The listing builds one solid part. Answer for the finished solid, in the listing's coordinates (mm). Round coordinates to 2 decimals unless told otherwise and drop trailing zeros. Loops run counter-clockwise (first coordinate to the right, second up) from the corner with the lowest first, then second, coordinate; pieces in that order, holes last. Notation, with made-up numbers: (-13.75, 78.25) -> (40.25, 78.25) arc R17 cw to (40.25, 93.25) -> close; hole circle Ø6 at (72.5, 43.5). An arc over 180 degrees is marked (long way). Use a Markdown table: item, result. Add a question column.
Q1. Given pin 1 Ø1.5 at (x, z) = (25.5, 2.5) entering from -Y; pin 2 Ø1.5 at (x, z) = (-12.5, 0.5) entering from -Y; pin 3 Ø0.9 at (y, z) = (0.5, 1) entering from +X; pin 4 Ø1.5 at (y, z) = (0, 1) entering from -X, each flat-ended and moving along its own axis, determine where each tip first touches the part or whether it passes through.
Q2. Consider line 1 (X direction, y = 0.25, z = 2.5); line 2 (X direction, y = 0.25, z = 3.8); line 3 (Z direction, x = -22, y = -5.75). Determine where each line is inside the solid, lowest interval first.
Q3. Section A-A on x = 0 is taken. Give the vertices of the cut face in (y, z), then the cut area to 3 significant figures.
Q4. Section C-C on z = 0.8 is taken. Give the vertices of the cut face in (x, y), then the cut area to 3 significant figures.
Q5. Section B-B on y = 0 is taken. Give the vertices of the cut face in (x, z), then the cut area to 4 significant figures.
Q6. Section D-D on x = 21.5 is taken. Give the vertices of the cut face in (y, z), then the cut area to 3 significant figures.
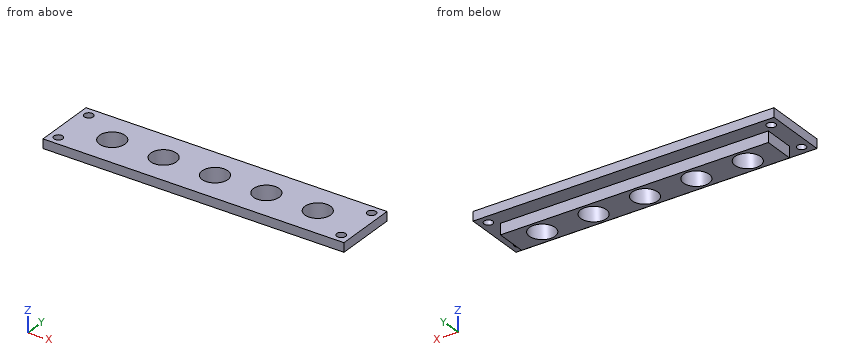
from build123d import *

# Parameters (mm, degrees)
SKETCH_1_W             = 73
SKETCH_1_H             = 8.4
EXTRUDE_1_DEPTH        = 3
SKETCH_2_W             = 82
SKETCH_2_H             = 17
EXTRUDE_2_DEPTH        = 2.5
SKETCH_3_R             = 3.5
CUT_EXTRUDE_1_DEPTH    = 10
PATTERN_LINEAR_1_COUNT = 3
PATTERN_LINEAR_1_PITCH = 14
PATTERN_LINEAR_2_COUNT = 3
PATTERN_LINEAR_2_PITCH = 14
SKETCH_4_R             = 1.2
CUT_EXTRUDE_4_DEPTH    = 6


with BuildPart() as part:
    # Эскиз1 → Бобышка-Вытянуть1 (new body)
    with BuildSketch(Plane.XY):
        Rectangle(SKETCH_1_W, SKETCH_1_H)
    extrude(amount=EXTRUDE_1_DEPTH)

    # Эскиз2 → Бобышка-Вытянуть2 (add)
    with BuildSketch(Plane.XY.offset(3)):
        Rectangle(SKETCH_2_W, SKETCH_2_H)
    extrude(amount=EXTRUDE_2_DEPTH)

    # Эскиз3 → Вырез-Вытянуть1 (cut)
    with BuildSketch(Plane(origin=(0, 0, 0), x_dir=(-1, 0, 0), z_dir=(0, 0, -1))):
        Circle(SKETCH_3_R)
    cut_extrude_1 = extrude(amount=-CUT_EXTRUDE_1_DEPTH, mode=Mode.SUBTRACT)

    # Линейный массив1: Вырез-Вытянуть1 ×3
    with Locations(*[(i * PATTERN_LINEAR_1_PITCH, 0, 0) for i in range(1, PATTERN_LINEAR_1_COUNT)]):
        add(cut_extrude_1, mode=Mode.SUBTRACT)

    # Линейный массив2: Вырез-Вытянуть1 ×3
    with Locations(*[(-i * PATTERN_LINEAR_2_PITCH, 0, 0) for i in range(1, PATTERN_LINEAR_2_COUNT)]):
        add(cut_extrude_1, mode=Mode.SUBTRACT)

    # Эскиз4 → Вырез-Вытянуть4 (cut)
    with BuildSketch(Plane.XY.offset(5.5)):
        with Locations((-38.524276055, 5.998931776)):
            Circle(SKETCH_4_R)
        with Locations((-38.524276055, -5.998931776)):
            Circle(SKETCH_4_R)
        with Locations((38.524276055, -5.998931776)):
            Circle(SKETCH_4_R)
        with Locations((38.524276055, 5.998931776)):
            Circle(SKETCH_4_R)
    extrude(amount=-CUT_EXTRUDE_4_DEPTH, mode=Mode.SUBTRACT)


solid = part.part
Checked values:
| question | item | result |
|---|---|---|
| 1 | pin 1 | stops at y = -8.5 |
| 1 | pin 2 | stops at y = -4.2 |
| 1 | pin 3 | stops at x = 36.5 |
| 1 | pin 4 | stops at x = -36.5 |
| 2 | line 1 | x = -36.5 to -31.49, -24.51 to -17.49, -10.51 to -3.49, 3.49 to 10.51, 17.49 to 24.51, 31.49 to 36.5 |
| 2 | line 2 | x = -41 to -31.49, -24.51 to -17.49, -10.51 to -3.49, 3.49 to 10.51, 17.49 to 24.51, 31.49 to 41 |
| 2 | line 3 | z = 3 to 5.5 |
| 3 | outline | (-8.5, 3) -> (-4.2, 3) -> (-4.2, 0) -> (-3.5, 0) -> (-3.5, 5.5) -> (-8.5, 5.5) -> close; (3.5, 0) -> (4.2, 0) -> (4.2, 3) -> (8.5, 3) -> (8.5, 5.5) -> (3.5, 5.5) -> close |
| 3 | area | 29.2 mm2 |
| 4 | outline | (-36.5, -4.2) -> (36.5, -4.2) -> (36.5, 4.2) -> (-36.5, 4.2) -> close; hole circle Ø7 at (-28, 0); hole circle Ø7 at (-14, 0); hole circle Ø7 at (0, 0); hole circle Ø7 at (14, 0); hole circle Ø7 at (28, 0) |
| 4 | area | 421 mm2 |
| 5 | outline | (-41, 3) -> (-36.5, 3) -> (-36.5, 0) -> (-31.5, 0) -> (-31.5, 5.5) -> (-41, 5.5) -> close; (-24.5, 0) -> (-17.5, 0) -> (-17.5, 5.5) -> (-24.5, 5.5) -> close; (-10.5, 0) -> (-3.5, 0) -> (-3.5, 5.5) -> (-10.5, 5.5) -> close; (3.5, 0) -> (10.5, 0) -> (10.5, 5.5) -> (3.5, 5.5) -> close; (17.5, 0) -> (24.5, 0) -> (24.5, 5.5) -> (17.5, 5.5) -> close; (31.5, 0) -> (36.5, 0) -> (36.5, 3) -> (41, 3) -> (41, 5.5) -> (31.5, 5.5) -> close |
| 5 | area | 231.5 mm2 |
| 6 | outline | (-8.5, 3) -> (-4.2, 3) -> (-4.2, 0) -> (4.2, 0) -> (4.2, 3) -> (8.5, 3) -> (8.5, 5.5) -> (-8.5, 5.5) -> close |
| 6 | area | 67.7 mm2 |
